Source: CAD feature listing. Evaluate the final solid. Frame: model axes, mm. Face numbers are marked on the shaded views. A direction names the side the tool comes from. Coordinates: 2 decimals unless noted, no trailing zeros. Write each loop counter-clockwise with the first axis right and the second up, starting at its lowest first coordinate (ties: lowest second). Pieces come first, ordered by that corner, then holes. Notation, with made-up numbers: (19, 24) - (57, 24) arc R25 cw to (57, 41) - close; hole circle Ø9 at (75.5, 24). An arc over 180 degrees is marked (long way). One line per item, written item: value.
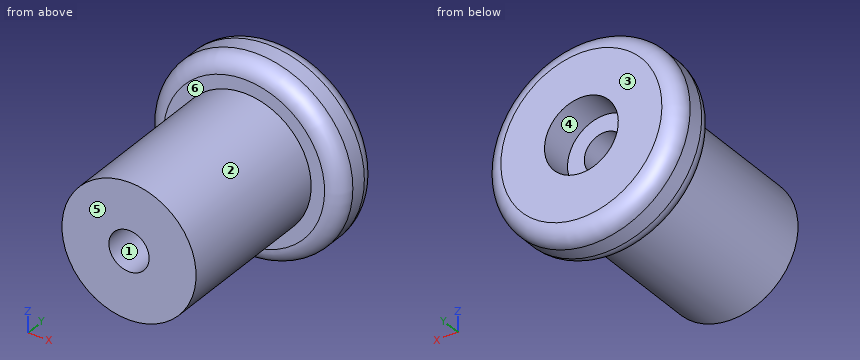
from build123d import *

# Parameters (mm, degrees)
SKETCH_1_R      = 4
EXTRUDE_1_DEPTH = 10
SKETCH_2_R      = 5.8
EXTRUDE_2_DEPTH = 3
FILLET_1_R      = 1


with BuildPart() as part:
    # 草图1 → 凸台-拉伸1 (new body)
    with BuildSketch(Plane(origin=(0, 0, 0), x_dir=(1, 0, 0), z_dir=(0, 1, 0))):
        with Locations(Location((0, 0, 0), (0, 0, 270))):
            Circle(SKETCH_1_R)
    extrude(amount=EXTRUDE_1_DEPTH)

    # 草图2 → 凸台-拉伸2 (add)
    with BuildSketch(Plane(origin=(0, 10, 0), x_dir=(1, 0, 0), z_dir=(0, 1, 0))):
        with Locations(Location((0, 0, 0), (0, 0, 270))):
            Circle(SKETCH_2_R)
    extrude(amount=EXTRUDE_2_DEPTH)

    # 草图4 → M2 凹头盖螺钉的柱形沉头孔1 (revolve, cut)
    with BuildSketch(Plane(origin=(0, 13, 0), x_dir=(0, 0, 1), z_dir=(1, 0, 0))):
        Polygon((0, 0), (0, 13), (1.2, 13), (1.2, 2), (2.2, 2), (2.2, 0), align=None)
    revolve(axis=Axis((0, 19.35, 0), (0, -1, 0)), mode=Mode.SUBTRACT)

    # 圆角1
    fillet_1_edges = [part.edges().sort_by_distance(p)[0] for p in [
        (0, 10, -5.8),
        (0, 13, -5.8),
    ]]
    fillet(fillet_1_edges, radius=FILLET_1_R)


solid = part.part
1) Material intervals for line 1 (X direction, y = 3.75, z = 0); line 2 (Z direction, x = -3.25, y = 11.75); line 3 (Y direction, x = 1.5, z = 1.25), sorted ascending.
Values found:
line 1: -4 to -1.2, 1.2 to 4
line 2: -4.8 to 4.8
line 3: 0 to 11
2) Contact query for flat-ended pins moving along their axis: P1, Ø1.5, axis at x = 1, y = 4.5, coming from the +Z side; P2, Ø2, axis at y = 2, z = -1, coming from the -X side; P3, Ø5, axis at x = -3, y = 10, coming from the -Z side. Output: stop coordinate, or through.
Values found:
P1: z = 3.99
P2: x = -4
P3: z = -5.76
3) Reachability of the marked faces 4, 5 and 6 from +Z, -Z, +X, -X, +Y, -Y: full face, straight path, thin tool, end or side. Return the list, or none.
Values found:
face 4: +Y
face 5: +Z, -Z, +X, -X, -Y
face 6: -Y
4) Section query A-A on x = 0. Output: boundary loops of the cut face in (y, z), then the cut area to 3 significant figures.
Values found:
outline: (0, -4) - (10, -4) - (10, -4.8) arc R1 ccw to (11, -5.8) - (12, -5.8) arc R1 ccw to (13, -4.8) - (13, -2.2) - (11, -2.2) - (11, -1.2) - (0, -1.2) - close; (0, 1.2) - (11, 1.2) - (11, 2.2) - (13, 2.2) - (13, 4.8) arc R1 ccw to (12, 5.8) - (11, 5.8) arc R1 ccw to (10, 4.8) - (10, 4) - (0, 4) - close
area: 78.7 mm2
5) Draft query along Z for the marked faces 1, 2 and 3. Return one class per face: released by +Z, released by -Z, zero draft, split by the parting line, or undercut.
Values found:
face 1: undercut
face 2: split by the parting line
face 3: zero draft
6) Section query C-C on y = 11.5. Output: boundary loops of the cut face in (x, z), then the cut area to 3 significant figures.
Values found:
outline: circle Ø11.6 at (0, 0); hole circle Ø4.4 at (0, 0)
area: 90.5 mm2
7) Section query D-D on y = 2. Output: boundary loops of the cut face in (x, z), then the cut area to 3 significant figures.
Values found:
outline: circle Ø8 at (0, 0); hole circle Ø2.4 at (0, 0)
area: 45.7 mm2
8) Section query B-B on z = 0. Output: boundary loops of the cut face in (x, y).
Values found:
outline: (-5.8, 11) arc R1 ccw to (-4.8, 10) - (-4, 10) - (-4, 0) - (-1.2, 0) - (-1.2, 11) - (-2.2, 11) - (-2.2, 13) - (-4.8, 13) arc R1 ccw to (-5.8, 12) - close; (1.2, 0) - (4, 0) - (4, 10) - (4.8, 10) arc R1 ccw to (5.8, 11) - (5.8, 12) arc R1 ccw to (4.8, 13) - (2.2, 13) - (2.2, 11) - (1.2, 11) - close
